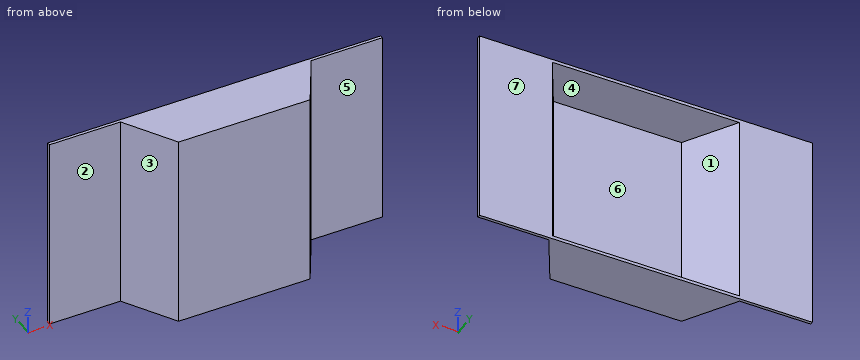
```python
from build123d import *

# Parameters (mm, degrees)
BOSS_EXTRUDE2_DEPTH = 381
SHELL1_START        = 6.096
SHELL1_DEPTH        = 368.808


# Read off the part's stored shape, not the designer's step: Shell1
with BuildPart() as part:
    # Sketch2 → Boss-Extrude2 (new body)
    with BuildSketch(Plane.XY):
        Polygon((-330.2, 101.6), (-185.65878735, 101.6), (185.65878735, 101.6), (330.2, 101.6), (330.2, 95.504), (189.178314591, 95.504), (130.519527241, -6.096), (-130.519527241, -6.096), (-189.178314591, 95.504), (-330.2, 95.504), align=None)
    extrude(amount=BOSS_EXTRUDE2_DEPTH)

    # Shell1 outline → Shell1 (cut)
    with BuildSketch(Plane.XY.offset(SHELL1_START)):
        Polygon((-185.65878735, 101.6), (-127, 0), (127, 0), (185.65878735, 101.6), align=None)
    extrude(amount=SHELL1_DEPTH, mode=Mode.SUBTRACT)


solid = part.part
```
Design review of the part built by this model. Coordinates are the model's own, in mm. Face numbers are marked on the shaded views. A direction names the side the tool comes from. Coordinates: 2 decimals unless noted, no trailing zeros. Write each loop counter-clockwise with the first axis right and the second up, starting at its lowest first coordinate (ties: lowest second). Pieces come first, ordered by that corner, then holes. Notation, with made-up numbers: M -32,21.25 L -14,21.25 A19 cw -14,26.25 Z; hole C 54.25,77 d8. An arc over 180 degrees is marked long. Answer as a JSON object with one key per item and string values.
Item 1: Insertion check: pin 1 Ø8 at (x, y) = (-132, 83) entering from -Z; pin 2 Ø3 at (y, z) = (53, 169) entering from +X; pin 3 Ø1 at (x, z) = (-152, 306) entering from -Y; pin 4 Ø1.5 at (y, z) = (15.5, 98) entering from +X. Each pin has a flat end and moves straight along its axis. Give the tip position at first contact, or say it passes through.
Outcome:
{"pin 1": "z = 0", "pin 2": "x = 165.5", "pin 3": "y = 30.24", "pin 4": "x = 143.42"}
Item 2: Draft analysis for pull direction X (two halves, no side actions). For the marked faces 1, 2, 3 and 4, state which applies: pulls with the +X half, pulls with the -X half, needs draft (parallel to the pull), parting line crosses it, or undercut.
Outcome:
{"face 1": "undercut", "face 2": "needs draft", "face 3": "pulls with the -X half", "face 4": "undercut"}
Item 3: Machinability: for the marked faces 5, 6 and 7, which of the approach directions +Z, -Z, +X, -X, +Y, -Y give a long, thin tool a straight path to every point of the face, cutting with its end or side? Answer none if there is none.
Outcome:
{"face 5": "+Z, -Z, +X, -Y", "face 6": "+Y", "face 7": "+Z, -Z, +X, -X, +Y"}
Item 4: Add section B-B, the plane x = 98.5. Give the boundary of the cut face in (y, z), and give its area (3 significant figures).
Outcome:
{"outline": "M -6.1,0 L 101.6,0 L 101.6,6.1 L 0,6.1 L 0,374.9 L 101.6,374.9 L 101.6,381 L -6.1,381 Z", "area": "3,560 mm²"}
Item 5: Add section C-C, the plane z = 83. Give the boundary of the cut face in (x, y), and give its area (3 significant figures).
Outcome:
{"outline": "M -330.2,95.5 L -189.18,95.5 L -130.52,-6.1 L 130.52,-6.1 L 189.18,95.5 L 330.2,95.5 L 330.2,101.6 L 185.66,101.6 L 127,0 L -127,0 L -185.66,101.6 L -330.2,101.6 Z", "area": "4,740 mm²"}
Item 6: Add section A-A, the plane y = 88.5. Give the boundary of the cut face in (x, z), and give its area (3 significant figures).
Outcome:
{"outline": "M -185.13,0 L 185.13,0 L 185.13,381 L -185.13,381 Z; hole M -178.1,6.1 L 178.1,6.1 L 178.1,374.9 L -178.1,374.9 Z", "area": "9,710 mm²"}
Item 7: Add section D-D, the plane y = 30. Give the boundary of the cut face in (x, z), and give its area (3 significant figures).
Outcome:
{"outline": "M -151.36,0 L 151.36,0 L 151.36,381 L -151.36,381 Z; hole M -144.32,6.1 L 144.32,6.1 L 144.32,374.9 L -144.32,374.9 Z", "area": "8,880 mm²"}
Item 8: Wall thickness on probe 1 along Z at (x, y) = (-72.5, 63); probe 2 along Y at (x, z) = (-223.5, 356); probe 3 along X at (y, z) = (65.5, 281): over which ranges is each line inside the solid? List them lowest first.
Outcome:
{"probe 1": "0 to 6.1, 374.9 to 381", "probe 2": "95.5 to 101.6", "probe 3": "-171.86 to -164.82, 164.82 to 171.86"}
